Study the drawing (mm; zero at the part's minimum x, y, z) and answer. A direction names the side the tool comes from. Round coordinates to 2 decimals unless told otherwise and drop trailing zeros. Write each loop counter-clockwise with the first axis right and the second up, starting at its lowest first coordinate (ties: lowest second). Pieces come first, ordered by that corner, then holes. Notation, with made-up numbers: M -33,54 L 4,54 A15 ccw 4,79 Z; hole C 58.25,32 d11. An arc over 180 degrees is marked long. Write each question's results on one line, items separated by ' | '.
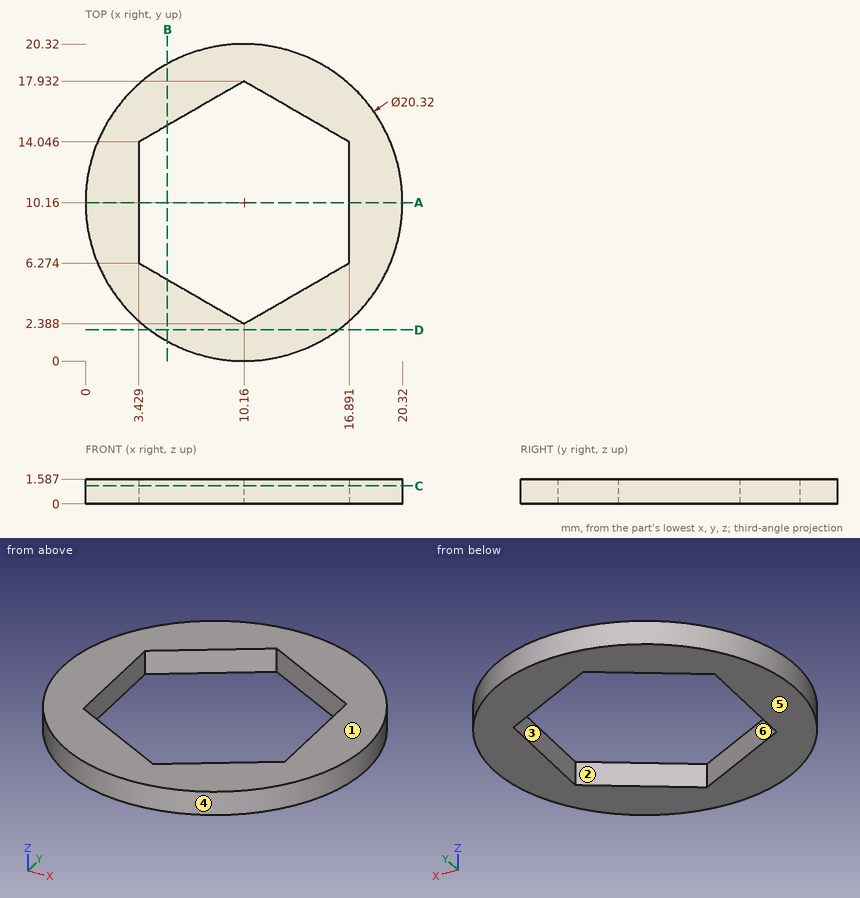
1) A tool of negligible diameter and unlimited length cuts with its end or side. For the marked faces 1 and 2, from which of +Z, -Z, +X, -X, +Y, -Y can it reach the whole face along a straight path? Write none if from no direction.
Return value:
face 1: +Z, +X, -X, +Y, -Y | face 2: +Z, -Z
2) Section D-D (y = 2) is taken. Determine the outline of the cut face in (x, z), then the cut area to 3 significant figures.
Return value:
outline: M 4.11,0 L 16.21,0 L 16.21,1.59 L 4.11,1.59 Z | area: 19.2 mm²
3) Section A-A (y = 10.16) is taken. Determine the outline of the cut face in (x, z), then the cut area to 3 significant figures.
Return value:
outline: M 0,0 L 3.43,0 L 3.43,1.59 L 0,1.59 Z; M 16.89,0 L 20.32,0 L 20.32,1.59 L 16.89,1.59 Z | area: 10.9 mm²
4) Find the intervals of material crossed by line 1 (X direction, y = 10, z = 0.1); line 2 (X direction, y = 11.5, z = 0.5); line 3 (Y direction, x = 8, z = 1.55) (1 decimal), in increasing order.
Return value:
line 1: 0 to 3.43, 16.89 to 20.32 | line 2: 0.09 to 3.43, 16.89 to 20.23 | line 3: 0.2 to 3.6, 16.7 to 20.1
5) Section C-C (z = 1.15) is taken. Determine the outline of the cut face in (x, y), then the cut area to 3 significant figures.
Return value:
outline: C 10.16,10.16 d20.32; hole M 3.43,6.27 L 10.16,2.39 L 16.89,6.27 L 16.89,14.05 L 10.16,17.93 L 3.43,14.05 Z | area: 167 mm²
6) Section B-B (x = 5.25) is taken. Determine the outline of the cut face in (y, z) (1 decimal).
Return value:
outline: M 1.3,0 L 5.2,0 L 5.2,1.6 L 1.3,1.6 Z; M 15.1,0 L 19.1,0 L 19.1,1.6 L 15.1,1.6 Z
7) The mould has two halves that part along X. Classify the marked faces 3, 4, 5 and 6: +X half, -X half, draft (parallel to the pull), parting line (faces both ways), or undercut.
Return value:
face 3: undercut | face 4: parting line | face 5: draft | face 6: undercut
8) Each of these flat-tipped pins is pushed along its axis until it touches: pin 1 (5 mm diameter, centred on x = 18.5, y = 17, fed in from -Z); pin 2 (1 mm diameter, centred on x = 7, y = 13.5, fed in from +Z). Where does it stop, or does it pass through?
Return value:
pin 1: z = 0 | pin 2: through
